The listing builds one solid part. Answer for the finished solid, in the listing's coordinates (mm). Give positions to 0.01 mm unless a question says otherwise; leave off trailing zeros. Order: outer loops, then holes, each group sorted by start corner. A loop starts at its lowest first (then second) coordinate and runs counter-clockwise, first axis right, second up. Notation, with made-up numbers: (-22.5, 55.25) - (-11.5, 55.25) arc R20 cw to (-11.5, 73.25) - close; hole circle Ø7 at (-10, 14). An arc over 180 degrees is marked (long way). Answer in a Markdown table with one row per item.
Autodesk Inventor part; units mm, degrees
ref_plane "YZ Plane" through (0, 0, 0) normal (1, 0, 0) x (0, 1, 0)
ref_plane "XZ Plane" through (0, 0, 0) normal (0, 1, 0) x (-1, 0, 0)
ref_plane "XY Plane" through (0, 0, 0) normal (0, 0, 1) x (1, 0, 0)
sketch "Boceto2" plane through (0, 0, 0) normal (0, 0, 1) x (1, 0, 0)
  line L0 (490, -50) -> (-510, -50)
  line L1 (-510, -50) -> (-510, 70)
  line L2 (-510, 70) -> (490, 70)
  line L3 (490, 70) -> (490, -50)
  line L4 (-510, 70) -> (-510, 30)
  line L5 (-510, 30) -> (490, 30)
  line L6 (-510, 30) -> (-510, -10)
  line L7 (-510, -10) -> (490, -10)
  point P0 (0, 0)
  dimension "d8" = 1000
  dimension "d14" = 120
  dimension "d15" = 40
  dimension "d16" = 40
extrude "Extrusión2" add sketch "Boceto2" along normal blind 3
sketch "Boceto4" plane through (0, 0, 3) normal (0, 0, 1) x (1, 0, 0)
  line L0 (-510, 30) -> (490, 30)
  line L1 (-510, -10) -> (490, -10)
  point P0 (0, 0)
bend part "Pieza de plegado2" radius 3 angle 90 line through (-510, 30, 3) along (1, 0, 0) centre toward (0, 0, 1) moving side (0, 1, 0) both sides yes
sketch "Boceto5" plane through (-510, 27.8787, 3.8787) normal (0, 0.7071068, 0.7071068) x (1, 0, 0)
  line L0 (0, -77.6438) -> (1000, -77.6438)
  line L1 (0, -77.6438) -> (0, -37.6438)
  line L2 (0, 0) -> (0, -77.6438)
  line L3 (0, -37.6438) -> (1000, -37.6438)
  line L4 (1000, -77.6438) -> (1000, 0)
  point P0 (510, -16.9706)
  dimension "d19" = 40
  dimension "d20" = 90
bend part "Pieza de plegado3" radius 3 angle 90 line through (-510, 1.2605, 30.4969) along (1, 0, 0) centre toward (0, 0.7071068, 0.7071068) moving side (0, 0.7071068, -0.7071068) both sides yes
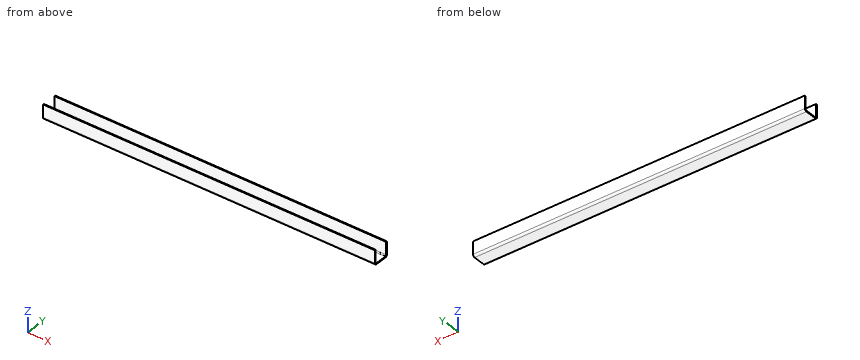
Item 1: Find section C-C on y = 19. Write down the section's boundary in (x, z).
Answer block:
| item | result |
|---|---|
| outline | (-510, 26.62) - (490, 26.62) - (490, 29.62) - (-510, 29.62) - close |
Item 2: Find section B-B on x = -328. Write down the section's boundary in (y, z).
Answer block:
| item | result |
|---|---|
| outline | (-2.62, 32.62) arc R6 ccw to (3.38, 26.62) - (38.67, 26.62) arc R6 ccw to (44.67, 32.62) - (44.67, 70.26) - (41.67, 70.26) - (41.67, 32.62) arc R3 cw to (38.67, 29.62) - (3.38, 29.62) arc R3 cw to (0.38, 32.62) - (0.38, 70.26) - (-2.62, 70.26) - close |
Item 3: Find section A-A on z = 41.5. Write down the section's boundary in (x, y).
Answer block:
| item | result |
|---|---|
| outline | (-510, -2.62) - (490, -2.62) - (490, 0.38) - (-510, 0.38) - close; (-510, 41.67) - (490, 41.67) - (490, 44.67) - (-510, 44.67) - close |
Item 4: Consider line 1 (Y direction, x = -333.5, z = 58.5); line 2 (Y direction, x = 201, z = 32); line 3 (Z direction, x = -455, y = 18). Determine where each line is inside the solid, lowest interval first.
Answer block:
| item | result |
|---|---|
| line 1 | -2.62 to 0.38, 41.67 to 44.67 |
| line 2 | -2.59 to 0.45, 41.61 to 44.64 |
| line 3 | 26.62 to 29.62 |
Item 5: Each of these flat-tipped pins is pushed along its axis until it touches: P1, Ø5, axis at x = -272.5, y = 11.5, coming from the +Z side; P2, Ø4, axis at x = -309.5, y = 3, coming from the +Z side; P3, Ø10, axis at x = -127, z = 31, coming from the +Y side. Where does it stop, or does it pass through?
Answer block:
| item | result |
|---|---|
| P1 | z = 29.62 |
| P2 | z = 30.79 |
| P3 | y = 44.67 |
